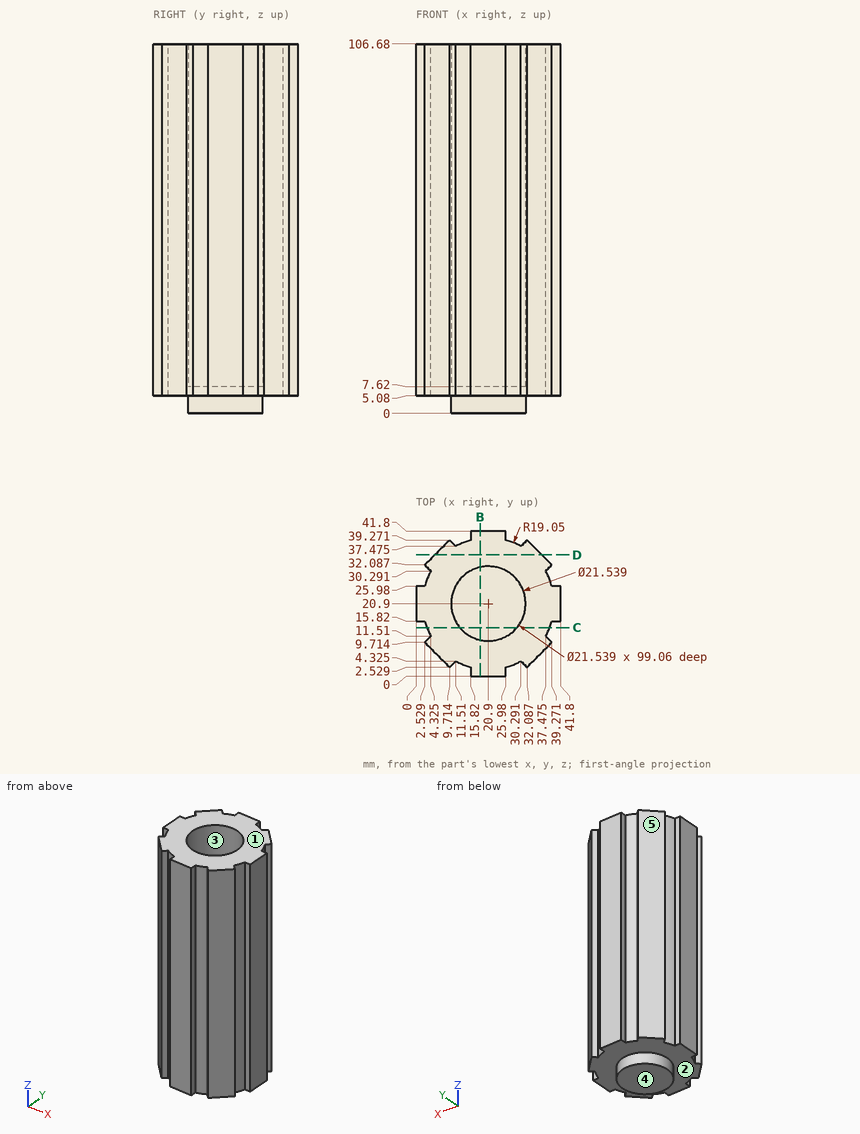
Answer from the drawing. Dimensions are ordinates in mm from the lowest x, y and z of the part. A direction names the side the tool comes from. Round coordinates to 2 decimals unless told otherwise and drop trailing zeros. Write each loop counter-clockwise with the first axis right and the second up, starting at its lowest first coordinate (ties: lowest second). Pieces come first, ordered by that corner, then holes.
1. Given pin 1 Ø3 at (y, z) = (40.5, 77) entering from +X; pin 2 Ø3 at (y, z) = (7.5, 42) entering from +X; pin 3 Ø5 at (x, z) = (36.5, 65.5) entering from +Y, each flat-ended and moving along its own axis, determine where each tip first touches the part or whether it passes through.
2. Which of the six approach directions +Z, -Z, +X, -X, +Y, -Y give full straight-line access (tool end or side, diameter ignored) to the marked faces 1 and 2?
3. The part is cut by section D-D, the plane y = 35. Determine the outline of the cut face in (x, z).
4. The part is cut by section C-C, the plane y = 14. Determine the outline of the cut face in (x, z).
5. The part is cut by section B-B, the plane x = 18.5. Determine the outline of the cut face in (y, z), then the cut area to 3 significant figures.
6. Determine the mould class of the marked faces 3, 4 and 5 for opening direction Y: pulls with the +Y half, pulls with the -Y half, needs draft (parallel to the pull), parting line crosses it, or undercut.
7. Straight lines are drawn through the part: L1, parallel to Y at x = 38, z = 97.5 (1 decimal); L2, parallel to Z at x = 29, y = 8.5; L3, parallel to Y at x = 23, z = 100.5. For each, find the intervals that lie inside material, in ascending order.
Values:
1. pin 1: stops at x = 32.36
1. pin 2: stops at x = 38.56
1. pin 3: stops at y = 37.36
2. face 1: +Z, +X, -X, +Y, -Y
2. face 2: -Z
3. outline: (5.44, 5.08) - (36.36, 5.08) - (36.36, 106.68) - (5.44, 106.68) - close
4. outline: (3.14, 5.08) - (12.63, 5.08) - (12.63, 0) - (29.17, 0) - (29.17, 5.08) - (38.66, 5.08) - (38.66, 106.68) - (29.17, 106.68) - (29.17, 7.62) - (12.63, 7.62) - (12.63, 106.68) - (3.14, 106.68) - close
5. outline: (0, 5.08) - (10.4, 5.08) - (10.4, 0) - (31.4, 0) - (31.4, 5.08) - (41.8, 5.08) - (41.8, 106.68) - (31.4, 106.68) - (31.4, 7.62) - (10.4, 7.62) - (10.4, 106.68) - (0, 106.68) - close
5. area: 2,270 mm2
6. face 3: undercut
6. face 4: needs draft
6. face 5: pulls with the +Y half
7. L1: y = 8.4 to 11, 12.5 to 29.3, 30.8 to 33.4
7. L2: z = 5.08 to 106.68
7. L3: y = 0 to 10.34, 31.46 to 41.8
